from build123d import *

# Parameters (mm, degrees)
F0_W      = 62.23
F0_H      = 12.7
F1_DEPTH  = 38.1
F3_DEPTH  = 5.08
F5_DEPTH  = 25.4
F6_R      = 9.525
F7_DEPTH  = 1.27
F8_R      = 6.985
F9_DEPTH  = 1.27
F10_R     = 3.81
F11_DEPTH = 1.27


with BuildPart() as f1:
    # F0 (on Front) → F1 (new body)
    with BuildSketch(Plane.XZ):
        with Locations((-31.115, 6.35)):
            Rectangle(F0_W, F0_H)
        with BuildLine():
            Line((0, 12.7), (0, 0))
            ThreePointArc((0, 0), (6.35, 6.35), (0, 12.7))
        make_face()
        with BuildLine():
            ThreePointArc((-62.23, 12.7), (-68.58, 6.35), (-62.23, 0))
            Line((-62.23, 0), (-62.23, 12.7))
        make_face()
    extrude(amount=F1_DEPTH)

    # F2 (on face) → F3 (cut)
    with BuildSketch(Plane.XZ.offset(38.1)):
        Polygon((-62.23, 1.814069), (0, 1.814069), (0, 11.170847), (-62.23, 11.466069), align=None)
    extrude(amount=-F3_DEPTH, mode=Mode.SUBTRACT)

    # F4 (on face) → F5 (cut)
    with BuildSketch(Plane.XZ.offset(33.02)):
        Polygon((-60.437147, 10.073616), (-60.437147, 3.723616), (-2.002486, 3.446399), (-2.002486, 9.796399), align=None)
    extrude(amount=-F5_DEPTH, mode=Mode.SUBTRACT)

    # F6 (on face) → F7 (cut)
    with BuildSketch(Plane(origin=(0, 0, 0), x_dir=(1, 0, 0), z_dir=(0, 0, -1))):
        with Locations((-50.196387, 16.022282)):
            Circle(F6_R)
        with Locations((-18.354639, 16.022282)):
            Circle(F6_R)
    extrude(amount=-F7_DEPTH, mode=Mode.SUBTRACT)

    # F8 (on face) → F9 (cut)
    with BuildSketch(Plane(origin=(0, 0, 1.27), x_dir=(1, 0, 0), z_dir=(0, 0, -1))):
        with Locations((-50.196387, 16.022282)):
            Circle(F8_R)
        with Locations((-18.557454, 16.427908)):
            Circle(F8_R)
    extrude(amount=-F9_DEPTH, mode=Mode.SUBTRACT)

    # F10 (on face) → F11 (cut)
    with BuildSketch(Plane(origin=(0, 0, 2.54), x_dir=(1, 0, 0), z_dir=(0, 0, -1))):
        with Locations((-50.196387, 16.022282)):
            Circle(F10_R)
        with Locations((-18.354639, 16.022282)):
            Circle(F10_R)
    extrude(amount=-F11_DEPTH, mode=Mode.SUBTRACT)


solid = f1.part
Build history of the part. All positions in model axes, mm. A direction names the side the tool comes from. Give positions to 0.01 mm unless a question says otherwise; leave off trailing zeros. Loops run counter-clockwise (first coordinate to the right, second up) from the corner with the lowest first, then second, coordinate; pieces in that order, holes last. Notation, with made-up numbers: (75.25, -23) -> (89.25, -23) arc R24 ccw to (89.25, 1) -> close; hole circle Ø9 at (12, 41). An arc over 180 degrees is marked (long way). Answer in a Markdown table with one row per item.
Item 1: Tool access for faces 1 (the flat face through (-32, -19, 0)), 2 (the cylindrical face through (-41.11, -18.88, 0.63)), 3 (the flat face through (-32, -36, 1.814)): list every direction of +Z, -Z, +X, -X, +Y, -Y with a clear straight run to the whole face (end or side of a thin tool).
Findings below:
| item | result |
|---|---|
| face 1 | -Z, +X, -X, +Y, -Y |
| face 2 | -Z |
| face 3 | -Y |
Item 2: Probe line 1 along X through (y, z) = (-13, 6.5); line 2 along Z through (x, y) = (-4, -14); line 3 along Y through (x, z) = (-48.5, 9.5). List the from-to ranges inside material, lowest first. Write a range as [from, to].
Findings below:
| item | result |
|---|---|
| line 1 | x = [-68.58, -60.44], [-2, 6.35] |
| line 2 | z = [0, 3.46], [9.81, 12.7] |
| line 3 | y = [-7.62, 0] |
Item 3: Slice it at A-A on x = -49.5. Write the cut outline in (y, z), plus the area to 3 significant figures.
Findings below:
| item | result |
|---|---|
| outline | (-38.1, 0) -> (-25.52, 0) -> (-25.52, 1.27) -> (-22.97, 1.27) -> (-22.97, 2.54) -> (-19.77, 2.54) -> (-19.77, 3.67) -> (-33.02, 3.67) -> (-33.02, 1.81) -> (-38.1, 1.81) -> close; (-38.1, 11.41) -> (-33.02, 11.41) -> (-33.02, 10.02) -> (-7.62, 10.02) -> (-7.62, 3.67) -> (-12.28, 3.67) -> (-12.28, 2.54) -> (-9.07, 2.54) -> (-9.07, 1.27) -> (-6.52, 1.27) -> (-6.52, 0) -> (0, 0) -> (0, 12.7) -> (-38.1, 12.7) -> close |
| area | 224 mm² |
Item 4: Slice it at D-D on x = -3. Write the cut outline in (y, z), plus the area to 3 significant figures.
Findings below:
| item | result |
|---|---|
| outline | (-38.1, 0) -> (0, 0) -> (0, 12.7) -> (-38.1, 12.7) -> (-38.1, 11.19) -> (-33.02, 11.19) -> (-33.02, 9.8) -> (-7.62, 9.8) -> (-7.62, 3.45) -> (-33.02, 3.45) -> (-33.02, 1.81) -> (-38.1, 1.81) -> close |
| area | 275 mm² |
Item 5: Flat gauge pins, fed straight in: P1, Ø6, axis at y = -5, z = 2.5, coming from the -X side; P2, Ø5, axis at x = -19.5, z = 6.5, coming from the -Y side; P3, Ø3.5, axis at x = -33, z = 5, coming from the -Y side. Where does each tip first touch, or does it go through?
Findings below:
| item | result |
|---|---|
| P1 | stops at x = -68.52 |
| P2 | stops at y = -7.62 |
| P3 | stops at y = -33.02 |
Item 6: Slice it at B-B on z = 6.35. Write the cut outline in (x, y).
Findings below:
| item | result |
|---|---|
| outline | (-68.58, -38.1) -> (-62.23, -38.1) -> (-62.23, -33.02) -> (-60.44, -33.02) -> (-60.44, -7.62) -> (-2, -7.62) -> (-2, -33.02) -> (0, -33.02) -> (0, -38.1) -> (6.35, -38.1) -> (6.35, 0) -> (-68.58, 0) -> close |
Item 7: Mould opens along Y. For faces 4 (the flat face through (-32, -38.1, 1)), 5 (the flat face through (-2.002, -20, 7)), 6 (the flat face through (-17, -20, 2.54)) say: pulls with the +Y half, pulls with the -Y half, needs draft (parallel to the pull), parting line crosses it, or undercut.
Findings below:
| item | result |
|---|---|
| face 4 | pulls with the -Y half |
| face 5 | needs draft |
| face 6 | undercut |
